Autodesk Inventor part; units mm, degrees
ref_plane "YZ Plane" through (0, 0, 0) normal (1, 0, 0) x (0, 1, 0)
ref_plane "XZ Plane" through (0, 0, 0) normal (0, 1, 0) x (-1, 0, 0)
ref_plane "XY Plane" through (0, 0, 0) normal (0, 0, 1) x (1, 0, 0)
sketch "Sketch1" plane through (0, 0, 0) normal (0, 1, 0) x (-1, 0, 0)
  line L0 (-63.5, 50.8) -> (63.5, 50.8)
  line L1 (63.5, 50.8) -> (63.5, -50.8)
  line L2 (63.5, -50.8) -> (-63.5, -50.8)
  line L3 (-63.5, -50.8) -> (-63.5, 50.8)
  line L4 (-63.5, 50.8) -> (63.5, -50.8) construction
  line L5 (63.5, 50.8) -> (-63.5, -50.8) construction
  point P0 (0, 0)
  dimension "d0" = 127
  dimension "d1" = 101.6
extrude "Extrusion1" add sketch "Sketch1" along normal blind 1.016
sketch "Sketch2" plane through (0, 1.016, 0) normal (0, 1, 0) x (1, 0, 0)
  line L0 (63.5, 50.8) -> (-63.5, 50.8)
  line L1 (63.5, -50.8) -> (-63.5, -50.8)
  line L2 (-63.5, -50.8) -> (-63.5, 50.8)
  line L3 (-63.5, 50.8) -> (63.5, 50.8)
  line L4 (63.5, 50.8) -> (63.5, -50.8)
  line L5 (63.5, -50.8) -> (-63.5, 50.8) construction
  line L6 (-63.5, -50.8) -> (63.5, 50.8) construction
  line L7 (62.992, -50.292) -> (-62.992, -50.292)
  line L8 (-62.992, -50.292) -> (-62.992, 50.292)
  line L9 (-62.992, 50.292) -> (62.992, 50.292)
  line L10 (62.992, 50.292) -> (62.992, -50.292)
  line L11 (62.992, -50.292) -> (-62.992, 50.292) construction
  line L12 (-62.992, -50.292) -> (62.992, 50.292) construction
  point P0 (0, 0)
  dimension "d4" = 125.984
  dimension "d5" = 100.584
extrude "Extrusion2" add sketch "Sketch2" along normal blind 50.8
sketch "Sketch3" plane through (-62.992, 1.016, -50.292) normal (0, 0, 1) x (1, 0, 0)
  line L0 (0, 0) -> (0, 50.8)
  circle A0 centre (37.592, 25.4) radius 2.0828
  circle A1 centre (88.392, 25.4) radius 2.0828
  point P0 (62.992, -1.016)
  dimension "d10" = 4.1656
  dimension "d12" = 4.1656
extrude "Extrusion3" cut sketch "Sketch3" against normal through all
sketch "Sketch4" plane through (0, 1.016, 0) normal (0, 1, 0) x (1, 0, 0)
  line L0 (50, -50) -> (-50, 50) construction
  line L1 (-50, -50) -> (50, 50) construction
  circle A0 centre (-43.65, -42.38) radius 1.4224
  circle A1 centre (-43.65, 42.38) radius 1.4224
  circle A2 centre (41.4402, 7.404) radius 1.4224
  point P0 (0, 0)
  dimension "d15" = 100
  dimension "d16" = 100
  dimension "d23" = 2.8448
  dimension "d24" = 2.8448
  dimension "d25" = 2.8448
extrude "Extrusion4" cut sketch "Sketch4" against normal through all
sketch "Sketch5" plane through (-62.992, 1.016, 50.292) normal (1, 0, 0) x (0, 0, -1)
  circle A0 centre (50.292, 19.05) radius 3.175
  point P0 (50.292, -1.016)
  dimension "d28" = 6.35
extrude "Extrusion5" cut sketch "Sketch5" against normal through all
sketch "Sketch6" plane through (62.992, 1.016, -50.292) normal (-1, 0, 0) x (0, 0, 1)
  line L0 (0, 0) -> (0, 50.8)
  line L1 (0, 19.05) -> (0.2921, 19.05)
  line L2 (0, 19.05) -> (0.2921, 19.05) construction
  line L3 (0.2921, 19.05) -> (20.1295, 19.05)
  line L4 (20.1295, 19.05) -> (31.2547, 19.05)
  line L5 (20.1295, 19.05) -> (31.2547, 19.05) construction
  line L6 (31.2547, 19.05) -> (66.1797, 19.05)
  line L7 (31.2547, 19.05) -> (66.1797, 19.05) construction
  line L8 (66.1797, 19.05) -> (79.6925, 19.05)
  line L9 (66.1797, 19.05) -> (79.6925, 19.05) construction
  circle A0 centre (20.1295, 19.05) radius 3.175
  circle A1 centre (31.2547, 19.05) radius 3.175
  circle A2 centre (66.1797, 19.05) radius 3.175
  circle A3 centre (79.6925, 19.05) radius 3.175
  point P0 (50.292, -1.016)
  dimension "d31" = 0.2921
  dimension "d32" = 0
  dimension "d33" = 19.8374
  dimension "d34" = 11.1252
  dimension "d35" = 0
  dimension "d36" = 34.925
  dimension "d37" = 0
  dimension "d38" = 13.5128
  dimension "d39" = 0
  dimension "d40" = 6.35
  dimension "d41" = 6.35
  dimension "d42" = 6.35
  dimension "d43" = 6.35
extrude "Extrusion6" cut sketch "Sketch6" against normal through all
equation "\"d29\" = d25"
properties part number "563-AC-1404-4xSplitter"
Geometry check sheet. Reference: the model listing, model coordinates, mm. A direction names the side the tool comes from. Round coordinates to 2 decimals unless told otherwise and drop trailing zeros. Loops run counter-clockwise (first coordinate to the right, second up) from the corner with the lowest first, then second, coordinate; pieces in that order, holes last. Notation, with made-up numbers: (-27, -22) - (14, -22) arc R15 cw to (14, 5) - close; hole circle Ø3 at (-30, 60.25). An arc over 180 degrees is marked (long way). Write item = value, one per line. Start each with the question number.
1. Thickness scan on line 1 (X direction, y = 30.5, z = -13); line 2 (Z direction, x = -35.5, y = 25); line 3 (X direction, y = 0.4, z = -42.38). Record the ranges inside material, lowest first.
2. Set-up check for faces 5 (the face through (63.242, 23.214, 15.474)), 6 (the face through (27.324, 25.618, -50.542)), 7 (the face through (-42.293, 0.515, 41.953)), 8 (the face through (-62.992, 26, 1)), 9 (the face through (-63.5, 26, 1)): record each of +Z, -Z, +X, -X, +Y, -Y from which the full face is reachable in a straight line by a thin tool's end or side.
3. Section check C-C on y = 12. Enter the section's corners in (x, z), then the cut area to 3 significant figures.
4. Section check D-D on z = 10.5. Enter the section's corners in (x, y).
5. Section check A-A on x = 25.4. Enter the section's corners in (y, z).
6. Section check B-B on z = 0. Enter the section's corners in (x, y).
7. Depth check by flat-ended pin: pin 1 (4 mm diameter, centred on y = 20.07, z = -30.16, fed in from +X); pin 2 (1.7 mm diameter, centred on x = -43.65, z = 42.38, fed in from -Y); pin 3 (12 mm diameter, centred on x = -39, z = 4.5, fed in from +Y). Enter the tip coordinate at first touch or a pass-through.
8. Mould release check, pull along X, two halves, no side actions. Record for faces 1 (the face through (63.5, 26, -1)), 2 (the face through (62.992, 26, -1)), 3 (the face through (1, 26, 50.8)), 4 (the face through (1, 1.016, 1)): released by +X, released by -X, zero draft, split by the parting line, or undercut.
Working result:
q1.line_1 = -63.5 to -62.99, 62.99 to 63.5
q1.line_2 = -50.8 to -50.29, 50.29 to 50.8
q1.line_3 = -63.5 to -45.07, -42.23 to 63.5
q2.face_5 = +X
q2.face_6 = -Z
q2.face_7 = +Y, -Y
q2.face_8 = +Y
q2.face_9 = +Z, -Z, -X, +Y, -Y
q3.outline = (-63.5, -50.8) - (63.5, -50.8) - (63.5, 50.8) - (-63.5, 50.8) - close; hole (-62.99, -50.29) - (62.99, -50.29) - (62.99, 50.29) - (-62.99, 50.29) - close
q3.area = 231 mm^2
q4.outline = (-63.5, 0) - (63.5, 0) - (63.5, 51.82) - (62.99, 51.82) - (62.99, 1.02) - (-62.99, 1.02) - (-62.99, 51.82) - (-63.5, 51.82) - close
q5.outline = (0, -50.8) - (24.33, -50.8) - (24.33, -50.29) - (1.02, -50.29) - (1.02, 50.29) - (51.82, 50.29) - (51.82, 50.8) - (0, 50.8) - close; (28.5, -50.8) - (51.82, -50.8) - (51.82, -50.29) - (28.5, -50.29) - close
q6.outline = (-63.5, 0) - (63.5, 0) - (63.5, 51.82) - (62.99, 51.82) - (62.99, 1.02) - (-62.99, 1.02) - (-62.99, 16.89) - (-63.5, 16.89) - close; (-63.5, 23.24) - (-62.99, 23.24) - (-62.99, 51.82) - (-63.5, 51.82) - close
q7.pin_1 = -62.99
q7.pin_2 = through
q7.pin_3 = 1.02
q8.face_1 = released by +X
q8.face_2 = undercut
q8.face_3 = zero draft
q8.face_4 = undercut
